Autodesk Inventor part; units mm, degrees
ref_plane "Start Plane" through (0, 0, 15) normal (0, 0, 1) x (1, 0, 0)
ref_plane "End Plane" through (0, 0, 70) normal (0, 0, 1) x (1, 0, 0)
ref_plane "Work Plane4" through (-130, 9, 15) normal (0, 0, -1) x (-1, 0, 0)
ref_plane "Start Plane" through (0, 0, 15) normal (0, 0, 1) x (1, 0, 0)
ref_plane "End Plane" through (0, 0, 70) normal (0, 0, 1) x (1, 0, 0)
sketch "Sketch" plane through (0, 0, 0) normal (0, 0, 1) x (1, 0, 0)
  line L0 (-15, -9) -> (-15, 9)
  line L1 (-9, 15) -> (9, 15)
  line L2 (15, 9) -> (15, -9)
  line L3 (9, -15) -> (-9, -15)
  arc A0 (-15, -9) -> (-9, -15) centre (-9, -9) ccw
  arc A1 (-9, 15) -> (-15, 9) centre (-9, 9) ccw
  arc A2 (15, 9) -> (9, 15) centre (9, 9) ccw
  arc A3 (9, -15) -> (15, -9) centre (9, -9) ccw
  arc A4 (-9, 12) -> (-12, 9) centre (-9, 9) ccw
  line L4 (-9, 12) -> (9, 12)
  arc A5 (12, 9) -> (9, 12) centre (9, 9) ccw
  line L5 (12, 9) -> (12, -9)
  arc A6 (9, -12) -> (12, -9) centre (9, -9) ccw
  line L6 (9, -12) -> (-9, -12)
  arc A7 (-12, -9) -> (-9, -12) centre (-9, -9) ccw
  line L7 (-12, -9) -> (-12, 9)
  line L8 (0, 22.7397) -> (0, -22.7397) construction
  line L9 (-22.7397, 0) -> (22.7397, 0) construction
  dimension "d7" = 6
  dimension "d10" = 30
  dimension "d11" = 30
  dimension "d12" = 3
  dimension "d15" = 15
  dimension "d16" = 15
extrude "Body" add sketch "Sketch" along normal up to surface (55 mm away) from surface at 15
sketch "Sketch3" plane through (0, 0, 0) normal (0, 0, 1) x (1, 0, 0)
  line L0 (0, 0) -> (10, 0)
ref_plane "Work Plane3" through (0, 0, 0) normal (0, -1, 0) x (1, 0, 0)
ref_plane "Work Plane4" through (-130, 9, 15) normal (0, 0, -1) x (-1, 0, 0)
split "Split1" plane through (-130, 9, 15) removes the side toward (0, 0, -1)
ref_plane "Work Plane5" through (0, 231, 70) normal (0, 0, 1) x (1, 0, 0)
split "Split2" plane through (0, 231, 70) removes the side toward (0, 0, 1)
sketch "Sketch4" plane through (0, 0, 0) normal (0, -1, 0) x (1, 0, 0)
  line L0 (-2, 15) -> (12, 15)
  line L1 (-2, 70) -> (12, 70)
  dimension "d18" = 55
equation "\"d7\" = G_IR"
equation "\"d10\" = G_H"
equation "\"d11\" = G_W"
equation "\"d12\" = G_T"
equation "\"d15\" = 0.5 * d10"
equation "\"d16\" = 0.5 * d11"
equation "\"d3\" = G_L"
equation "\"G_W\" = 30"
equation "\"G_H\" = 30"
equation "\"G_T\" = 3"
equation "\"G_IR\" = 6"
equation "\"G_L\" = d18"
equation "\"G_OFFSET_START\" = -15"
equation "\"G_OFFSET_END\" = -15"
equation "\"d13\" = -G_OFFSET_START"
equation "\"B_L\" = 85"
properties part number "DIN EN 10219-2 - 30 x 30 x 3  - 55" material "Steel, Mild"
Can you work these out from the model? Positions are in its coordinate system, mm. A direction names the side the tool comes from. Coordinates: 2 decimals unless noted, no trailing zeros. Write each loop counter-clockwise with the first axis right and the second up, starting at its lowest first coordinate (ties: lowest second). Pieces come first, ordered by that corner, then holes. Notation, with made-up numbers: (69, -32) -> (113, -32) arc R16 ccw to (113, -10) -> close; hole circle Ø1 at (11.25, -15). An arc over 180 degrees is marked (long way). Write item = value, one per line.
(1) Imagine slicing it at A-A (y = -8.25). Please give me the cut outline in (x, z).
Verdict:
outline = (-15, 15) -> (-12, 15) -> (-12, 70) -> (-15, 70) -> close; (12, 15) -> (15, 15) -> (15, 70) -> (12, 70) -> close
(2) If I drill on probe 1 along Y at (x, z) = (-8.25, 42); probe 2 along X at (y, z) = (-11, 64), over which ranges is the centre line in solid material (lowest first)?
Verdict:
probe_1 = -15 to -12, 12 to 15
probe_2 = -14.66 to -11.24, 11.24 to 14.66
(3) Imagine slicing it at B-B (z = 21). Please give me the cut outline in (x, y).
Verdict:
outline = (-15, -9) arc R6 ccw to (-9, -15) -> (9, -15) arc R6 ccw to (15, -9) -> (15, 9) arc R6 ccw to (9, 15) -> (-9, 15) arc R6 ccw to (-15, 9) -> close; hole (-12, -9) arc R3 ccw to (-9, -12) -> (9, -12) arc R3 ccw to (12, -9) -> (12, 9) arc R3 ccw to (9, 12) -> (-9, 12) arc R3 ccw to (-12, 9) -> close
(4) On a 3-axis mill with a long thin cutter (end or side, diameter ignored), from which of +Z, -Z, +X, -X, +Y, -Y can I reach the whole of each face in a straight line? I mean faces 4 (the face through (0, -12, 42)), 5 (the face through (-13.196, -13.289, 42.115)). Say none if no direction works.
Verdict:
face_4 = +Z, -Z
face_5 = +Z, -Z, -X, -Y
(5) Thinking about a two-plate mould opening in Y: for faces 1 (the face through (-11.14, 11.1, 42.11)), 2 (the face through (13.196, 13.289, 42.115)), 3 (the face through (-12.3, 0.1, 15)), which applies, +Y half, -Y half, draft (parallel to the pull), parting line (faces both ways), or undercut?
Verdict:
face_1 = undercut
face_2 = +Y half
face_3 = draft
